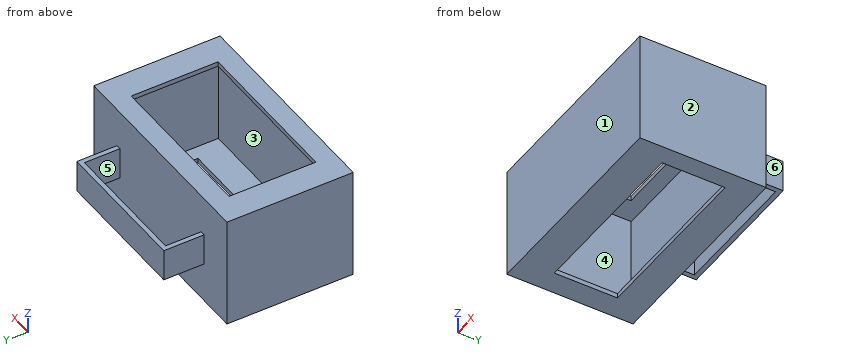
from build123d import *

# Parameters (mm, degrees)
SKETCH1_W           = 136
SKETCH1_H           = 71
BOSS_EXTRUDE2_DEPTH = 80
SHELL5_T            = -3
SKETCH2_W           = 130
SKETCH2_H           = 3
BOSS_EXTRUDE3_DEPTH = 74
BOSS_EXTRUDE4_DEPTH = 10.16
SKETCH7_W           = 100
SKETCH7_H           = 55
CUT_EXTRUDE1_DEPTH  = 10
SKETCH8_W           = 110
SKETCH8_H           = 40
CUT_EXTRUDE2_DEPTH  = 10


with BuildPart() as part:
    # Sketch1 → Boss-Extrude2 (new body)
    with BuildSketch(Plane(origin=(0, 0, 0), x_dir=(1, 0, 0), z_dir=(0, 1, 0))):
        Rectangle(SKETCH1_W, SKETCH1_H)
    extrude(amount=BOSS_EXTRUDE2_DEPTH)

    # Shell5
    shell5_openings = [part.faces().sort_by_distance(p)[0] for p in [
        (0, 40, 35.5),
    ]]
    offset(amount=SHELL5_T, openings=shell5_openings, kind=Kind.INTERSECTION)

    # Sketch2 → Boss-Extrude3 (add)
    with BuildSketch(Plane(origin=(0, 3, 0), x_dir=(1, 0, 0), z_dir=(0, 1, 0))):
        with Locations((0, -34)):
            Rectangle(SKETCH2_W, SKETCH2_H)
    extrude(amount=BOSS_EXTRUDE3_DEPTH)

    # Sketch4 → Boss-Extrude4 (add, symmetric)
    with BuildSketch(Plane.XY):
        Polygon((-44.45, 80), (-44.45, 105.4), (44.45, 105.4), (44.45, 80), (41.45, 80), (41.45, 102.4), (-41.45, 102.4), (-41.45, 80), align=None)
    extrude(amount=BOSS_EXTRUDE4_DEPTH, both=True)

    # Sketch7 → Cut-Extrude1 (cut)
    with BuildSketch(Plane.XY.offset(35.5)):
        with Locations((0, 40)):
            Rectangle(SKETCH7_W, SKETCH7_H)
    extrude(amount=-CUT_EXTRUDE1_DEPTH, mode=Mode.SUBTRACT)

    # Sketch8 → Cut-Extrude2 (cut)
    with BuildSketch(Plane(origin=(0, 0, -35.5), x_dir=(-1, 0, 0), z_dir=(0, 0, -1))):
        with Locations((-1.324990804, 41.229977006)):
            Rectangle(SKETCH8_W, SKETCH8_H)
    extrude(amount=-CUT_EXTRUDE2_DEPTH, mode=Mode.SUBTRACT)


solid = part.part
The listing builds one solid part. Answer for the finished solid, in the listing's coordinates (mm). Face numbers are marked on the shaded views. A direction names the side the tool comes from. Give positions to 0.01 mm unless a question says otherwise; leave off trailing zeros. Write each loop counter-clockwise with the first axis right and the second up, starting at its lowest first coordinate (ties: lowest second). Pieces come first, ordered by that corner, then holes.
1) Section D-D (x = 3) is taken. Write down the section's boundary in (y, z).
2) Section B-B (x = -47.5) is taken. Write down the section's boundary in (y, z), and give its area (3 significant figures).
3) Section A-A (y = 95) is taken. Write down the section's boundary in (x, z), and give its area (3 significant figures).
4) Given P1, Ø12.5, axis at x = 18, y = 93.5, coming from the -Z side; P2, Ø20.5, axis at x = -19, y = 96, coming from the +Z side; P3, Ø0.9, axis at x = 19.5, z = -34, coming from the +Y side; P4, Ø22.5, axis at y = 92.5, z = -1.5, coming from the +X side, each flat-ended and moving along its own axis, determine where each tip first touches the part or whether it passes through.
5) A tool of negligible diameter and unlimited length cuts with its end or side. For the marked faces 4, 5 and 6, from which of +Z, -Z, +X, -X, +Y, -Y can it reach the whole face along a straight path? Write none if from no direction.
6) Find the intervals of material crossed by L1, parallel to Y at x = 23, z = -8; L2, parallel to Y at x = -42.5, z = -17.5; L3, parallel to X at y = 32, z = -23, in increasing order.
7) For a pull along X with two mould halves and no side action, classify the marked faces 1, 2 and 3 as pulls with the +X half, pulls with the -X half, needs draft (parallel to the pull), parting line crosses it, or undercut.
8) Section C-C (z = 16) is taken. Write down the section's boundary in (x, y).
Response:
1. outline: (0, -35.5) - (21.23, -35.5) - (21.23, -32.5) - (3, -32.5) - (3, 32.5) - (12.5, 32.5) - (12.5, 35.5) - (0, 35.5) - close; (61.23, -35.5) - (80, -35.5) - (80, 35.5) - (67.5, 35.5) - (67.5, 32.5) - (77, 32.5) - (77, -32.5) - (61.23, -32.5) - close; (102.4, -10.16) - (105.4, -10.16) - (105.4, 10.16) - (102.4, 10.16) - close
2. outline: (0, -35.5) - (21.23, -35.5) - (21.23, -32.5) - (3, -32.5) - (3, 32.5) - (12.5, 32.5) - (12.5, 35.5) - (0, 35.5) - close; (61.23, -35.5) - (80, -35.5) - (80, 35.5) - (67.5, 35.5) - (67.5, 32.5) - (77, 32.5) - (77, -32.5) - (61.23, -32.5) - close
2. area: 585 mm2
3. outline: (-44.45, -10.16) - (-41.45, -10.16) - (-41.45, 10.16) - (-44.45, 10.16) - close; (41.45, -10.16) - (44.45, -10.16) - (44.45, 10.16) - (41.45, 10.16) - close
3. area: 122 mm2
4. P1: passes through
4. P2: stops at z = 10.16
4. P3: stops at y = 80
4. P4: stops at x = 44.45
5. face 4: none
5. face 5: +Z, -Z
5. face 6: +Z, -Z, +X, +Y
6. L1: y = 0 to 3, 77 to 80, 102.4 to 105.4
6. L2: y = 0 to 3, 77 to 80
6. L3: x = -68 to -65, 65 to 68
7. face 1: needs draft
7. face 2: pulls with the +X half
7. face 3: undercut
8. outline: (-68, 0) - (68, 0) - (68, 80) - (-68, 80) - close; hole (-65, 3) - (65, 3) - (65, 77) - (-65, 77) - close
